Verification items for this drawing (mm, ordinates from the low corner). A direction names the side the tool comes from. Coordinates: 2 decimals unless noted, no trailing zeros. Order: outer loops, then holes, each group sorted by start corner. A loop starts at its lowest first (then second) coordinate and runs counter-clockwise, first axis right, second up. Notation, with made-up numbers: (-12.5, 82) - (34.5, 82) arc R13 ccw to (34.5, 101) - close; hole circle Ø11 at (60, 40). An arc over 180 degrees is marked (long way). Use CSV: the item, a comma, the result in double quotes. Start each with the question number.
1) Sectioned sample at C-C, the plane y = 21. Record the cut outline in (x, z).
2) Depth check by flat-ended pin: P1, Ø4, axis at x = 25, y = 30, coming from the +Z side. Enter the tip coordinate at first touch or a pass-through.
3) Sectioned sample at B-B, the plane z = 23. Record the cut outline in (x, y), and give its area (3 significant figures).
4) Tool access check on the marked faces 4 and 5. Record the directions out of +Z, -Z, +X, -X, +Y, -Y that give a thin tool (end or side, any length) a straight path to the whole face; none if there is none.
5) Sectioned sample at D-D, the plane y = 38. Record the cut outline in (x, z), and give its area (3 significant figures).
6) Sectioned sample at A-A, the plane x = 38. Record the cut outline in (y, z).
7) Draft check along X on the marked faces 1, 2 and 3. Enter one of: released by +X, released by -X, zero draft, split by the parting line, or undercut.
8) Thickness scan on probe 1 along X at (y, z) = (14, 4); probe 2 along Y at (x, z) = (56.5, 10.5); probe 3 along Y at (x, z) = (38, 0.9). Record the ranges inside material, lowest first. Write a range as [from, to].
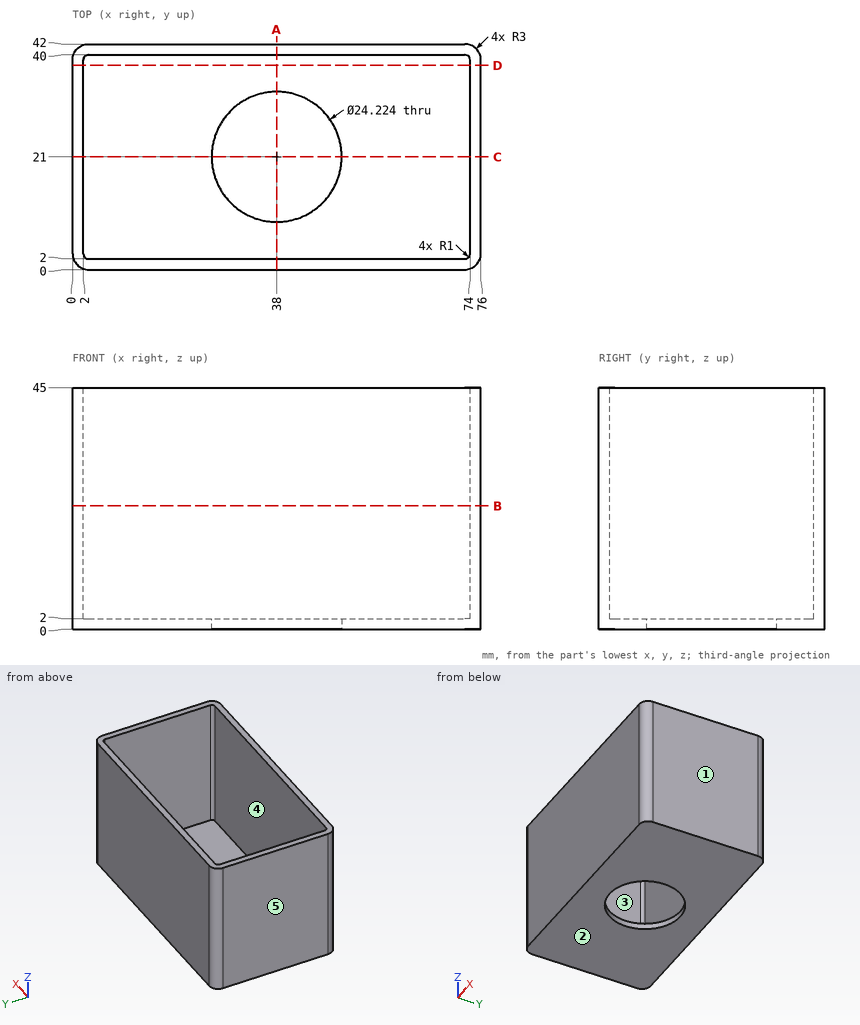
Evaluation:
1,outline,"(0, 0) - (25.89, 0) - (25.89, 2) - (2, 2) - (2, 45) - (0, 45) - close; (50.11, 0) - (76, 0) - (76, 45) - (74, 45) - (74, 2) - (50.11, 2) - close"
2,P1,"z = 2"
3,outline,"(0, 3) arc R3 ccw to (3, 0) - (73, 0) arc R3 ccw to (76, 3) - (76, 39) arc R3 ccw to (73, 42) - (3, 42) arc R3 ccw to (0, 39) - close; hole (2, 3) arc R1 ccw to (3, 2) - (73, 2) arc R1 ccw to (74, 3) - (74, 39) arc R1 ccw to (73, 40) - (3, 40) arc R1 ccw to (2, 39) - close"
3,area,"449 mm²"
4,face 4,"+Z"
4,face 5,"+Z, -Z, -X, +Y, -Y"
5,outline,"(0, 0) - (76, 0) - (76, 45) - (74, 45) - (74, 2) - (2, 2) - (2, 45) - (0, 45) - close"
5,area,"324 mm²"
6,outline,"(0, 0) - (8.89, 0) - (8.89, 2) - (2, 2) - (2, 45) - (0, 45) - close; (33.11, 0) - (42, 0) - (42, 45) - (40, 45) - (40, 2) - (33.11, 2) - close"
7,face 1,"released by +X"
7,face 2,"zero draft"
7,face 3,"undercut"
8,probe 1,"[0, 2], [74, 76]"
8,probe 2,"[0, 2], [40, 42]"
8,probe 3,"[0, 8.89], [33.11, 42]"
